Drawing for the job (mm, zero at the part's lowest x, y, z). A direction names the side the tool comes from. Round coordinates to 2 decimals unless told otherwise and drop trailing zeros. Order: outer loops, then holes, each group sorted by start corner. A loop starts at its lowest first (then second) coordinate and runs counter-clockwise, first axis right, second up. Notation, with made-up numbers: M 78,5 L 125,5 A22 cw 125,13 Z; hole C 55.5,62 d7. An arc over 180 degrees is marked long. One line per item, written item: value. Start each with the question number.
Item 1: Pin check, flat tips, straight feed: pin 1 (1.5 mm diameter, centred on x = 20, z = 17, fed in from -Y); pin 2 (2 mm diameter, centred on y = 10.5, z = 11, fed in from +X). Stop position of each tip, or through.
Item 2: Band-saw the part on C-C, the plane z = 12.7. Write the cut outline in (x, y) (3 decimals).
Item 3: Probe L1, parallel to Z at x = 12.7, y = 14.65 (3 decimals); L2, parallel to Y at x = 6.25, z = 14.25. List the from-to ranges inside material, lowest first.
Item 4: Tool access for the marked faces 5, 6 and 7: list every direction of +Z, -Z, +X, -X, +Y, -Y with a clear straight run to the whole face (end or side of a thin tool).
Item 5: Band-saw the part on B-B, the plane x = 23. Write the cut outline in (y, z).
Item 6: Band-saw the part on D-D, the plane x = 12.7. Write the cut outline in (y, z) (3 decimals).
Item 7: Band-saw the part on A-A, the plane z = 19.5. Write the cut outline in (x, y), then the cut area to 3 significant figures.
Item 8: Two-plate mould, pull along Y, no slides. Class the marked faces 1, 2, 3 and 4: +Y half, -Y half, draft (parallel to the pull), parting line (faces both ways), or undercut.
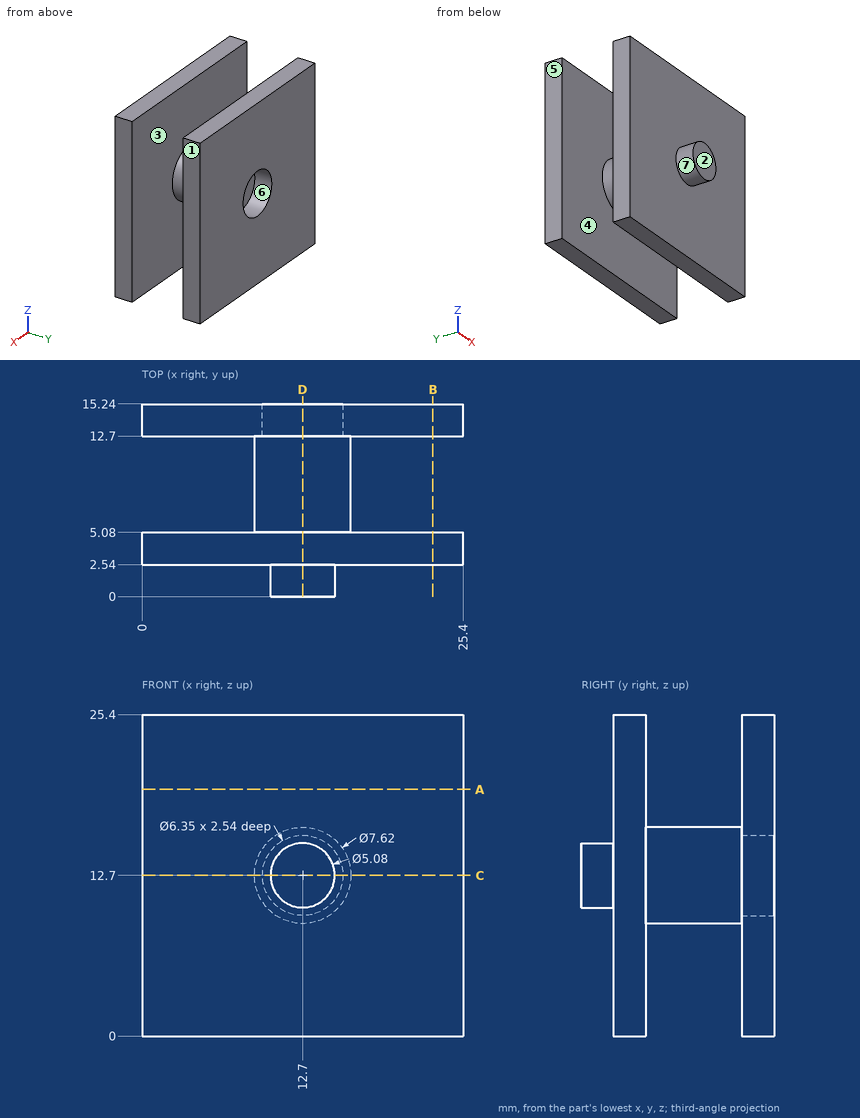
Output:
1. pin 1: stops at y = 2.54
1. pin 2: stops at x = 16.45
2. outline: M 0,2.54 L 10.16,2.54 L 10.16,0 L 15.24,0 L 15.24,2.54 L 25.4,2.54 L 25.4,5.08 L 16.51,5.08 L 16.51,12.7 L 25.4,12.7 L 25.4,15.24 L 15.875,15.24 L 15.875,12.7 L 9.525,12.7 L 9.525,15.24 L 0,15.24 L 0,12.7 L 8.89,12.7 L 8.89,5.08 L 0,5.08 Z
3. L1: z = 0 to 9.525, 15.875 to 25.4
3. L2: y = 2.54 to 5.08, 12.7 to 15.24
4. face 5: +Z, -Z, -X, +Y, -Y
4. face 6: +Y
4. face 7: -Y
5. outline: M 2.54,0 L 5.08,0 L 5.08,25.4 L 2.54,25.4 Z; M 12.7,0 L 15.24,0 L 15.24,25.4 L 12.7,25.4 Z
6. outline: M 0,10.16 L 2.54,10.16 L 2.54,0 L 5.08,0 L 5.08,8.89 L 12.7,8.89 L 12.7,0 L 15.24,0 L 15.24,9.525 L 12.7,9.525 L 12.7,15.875 L 15.24,15.875 L 15.24,25.4 L 12.7,25.4 L 12.7,16.51 L 5.08,16.51 L 5.08,25.4 L 2.54,25.4 L 2.54,15.24 L 0,15.24 Z
7. outline: M 0,2.54 L 25.4,2.54 L 25.4,5.08 L 0,5.08 Z; M 0,12.7 L 25.4,12.7 L 25.4,15.24 L 0,15.24 Z
7. area: 129 mm²
8. face 1: draft
8. face 2: -Y half
8. face 3: undercut
8. face 4: undercut
